Design review of the part shown in the three views and the two pictorial views. Dimensions are in mm from the part's minimum x, y and z. Coordinates: 2 decimals unless noted, no trailing zeros. Write each loop counter-clockwise with the first axis right and the second up, starting at its lowest first coordinate (ties: lowest second). Pieces come first, ordered by that corner, then holes. Notation, with made-up numbers: (19, 71) -> (23, 71) arc R6 ccw to (23, 79) -> close; hole circle Ø9 at (68.5, 3.25). An arc over 180 degrees is marked (long way). Write each question's results on one line, items separated by ' | '.
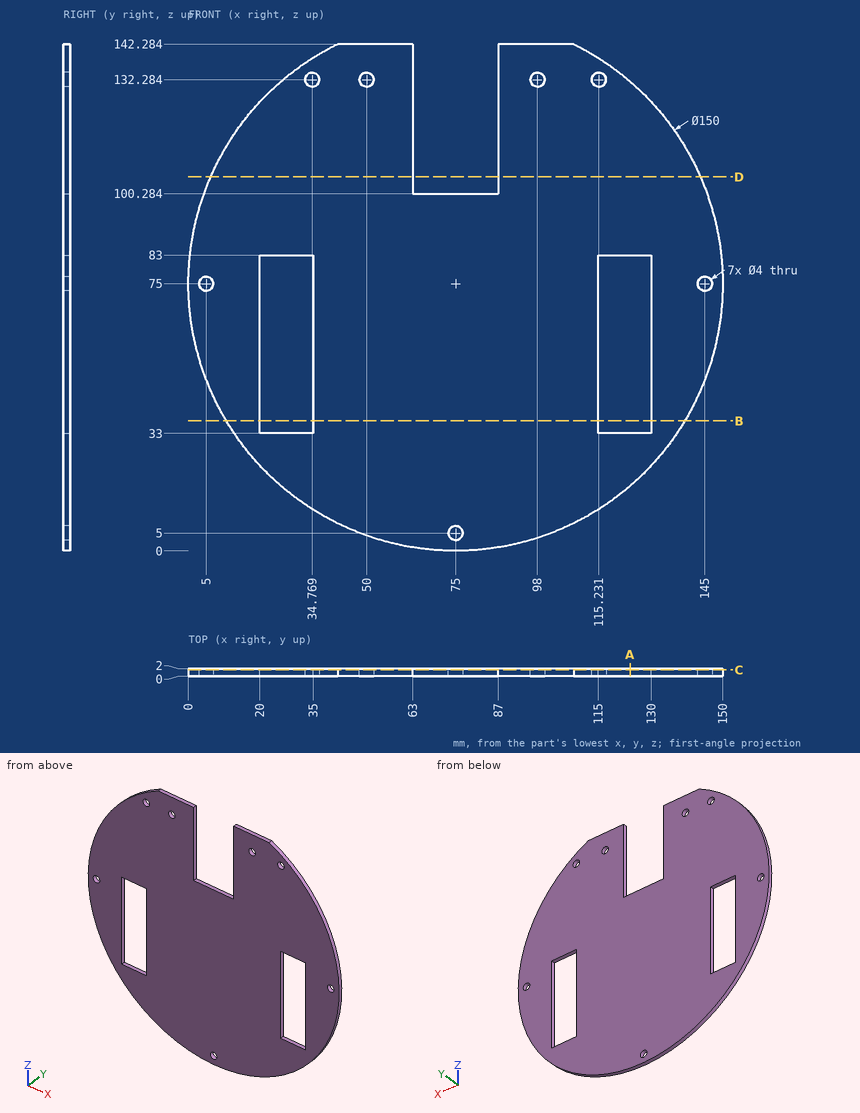
Q1. Add section B-B (z = 36.5). Write out the cut boundary in (x, y).
Solution:
outline: (10.64, 0) -> (20, 0) -> (20, 2) -> (10.64, 2) -> close; (35, 0) -> (115, 0) -> (115, 2) -> (35, 2) -> close; (130, 0) -> (139.36, 0) -> (139.36, 2) -> (130, 2) -> close
Q2. For line 1 (X direction, y = 1.2, z = 68.5); line 2 (X direction, y = 0.3, z = 66); line 3 (X direction, y = 0.4, z = 102.5), list the stretches that pass through material, from the lowest coordinate up. Write a range as from..to.
Solution:
line 1: 0.28..20, 35..115, 130..149.72 | line 2: 0.54..20, 35..115, 130..149.46 | line 3: 5.22..63, 87..144.78
Q3. Add section C-C (y = 1.7). Count the separate pieces of the cut face and the enclosed holes in it, plus the area to 3 significant figures.
Solution:
separate pieces: 1 | enclosed holes: 9 | area: 14,700 mm²
Q4. Add section D-D (z = 105). Write out the cut boundary in (x, y).
Solution:
outline: (6.26, 0) -> (63, 0) -> (63, 2) -> (6.26, 2) -> close; (87, 0) -> (143.74, 0) -> (143.74, 2) -> (87, 2) -> close
Q5. Clearance check with flat-ended pins moving along their axes: P1, Ø6.5, axis at x = 115.23, z = 132.28, coming from the +Y side; P2, Ø2.5, axis at x = 75, z = 5, coming from the +Y side; P3, Ø1, axis at x = 26, y = 1, coming from the +Z side; P4, Ø0.6, axis at x = 78, y = 0.5, coming from the +Z side. State where each tip first meets the part, or that it passes through.
Solution:
P1: y = 2 | P2: through | P3: z = 132.21 | P4: z = 100.28
Q6. Add section A-A (x = 124). Write out the cut boundary in (y, z).
Solution:
outline: (0, 18.22) -> (2, 18.22) -> (2, 33) -> (0, 33) -> close; (0, 83) -> (2, 83) -> (2, 131.78) -> (0, 131.78) -> close
